For this review, take the finished solid that the model builds, in its own axes (mm). Round coordinates to 2 decimals unless told otherwise and drop trailing zeros. Loops run counter-clockwise (first coordinate to the right, second up) from the corner with the lowest first, then second, coordinate; pieces in that order, holes last.
1. Clearance check with flat-ended pins moving along their axes: pin 1 Ø7 at (x, y) = (59, 19) entering from +Z; pin 2 Ø1 at (x, z) = (68, -2.5) entering from +Y; pin 3 Ø3 at (y, z) = (51.5, -2.5) entering from +X. State where each tip first meets the part, or that it passes through.
2. Consider section A-A on x = 19. State the section outline as (y, z) points, then the cut area to 3 significant figures.
3. To check wall thickness, follow line 1 along Y through (x, z) = (19, 1.15); line 2 along Y through (x, z) = (16.5, 1.25); line 3 along X through (y, z) = (59.5, -1). State the ranges of each line that lie inside material, in increasing order.
4. Consider section B-B on z = 0.25. State the section outline as (x, y) points, then the cut area to 3 significant figures.
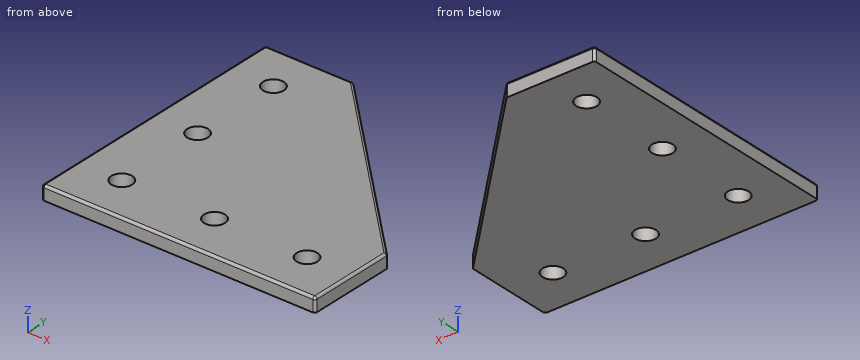
from build123d import *

# Parameters (mm, degrees)
SKETCH1_R           = 4.5
BOSS_EXTRUDE1_DEPTH = 3
FILLET1_R           = 1


with BuildPart() as part:
    # Sketch1 → Boss-Extrude1 (new, symmetric)
    with BuildSketch(Plane.XY):
        Polygon((0, 0), (0, 118), (38, 118), (118, 38), (118, 0), align=None)
        with Locations((19, 19)):
            Circle(SKETCH1_R, mode=Mode.SUBTRACT)
        with Locations((59, 19)):
            Circle(SKETCH1_R, mode=Mode.SUBTRACT)
        with Locations((99, 19)):
            Circle(SKETCH1_R, mode=Mode.SUBTRACT)
        with Locations((19, 59)):
            Circle(SKETCH1_R, mode=Mode.SUBTRACT)
        with Locations((19, 99)):
            Circle(SKETCH1_R, mode=Mode.SUBTRACT)
    extrude(amount=BOSS_EXTRUDE1_DEPTH, both=True)

    # Fillet1
    fillet1_edges = [part.edges().sort_by_distance(p)[0] for p in [
        (78, 78, 3),
        (19, 118, 3),
        (0, 59, 3),
        (59, 0, 3),
        (118, 19, 3),
        (0, 0, 0),
        (0, 118, 0),
        (38, 118, 0),
        (118, 38, 0),
        (118, 0, 0),
    ]]
    fillet(fillet1_edges, radius=FILLET1_R)


solid = part.part
Resolved:
1. pin 1: passes through
1. pin 2: stops at y = 88.5
1. pin 3: stops at x = 106
2. outline: (0, -3) - (14.5, -3) - (14.5, 3) - (1, 3) arc R1 ccw to (0, 2) - close; (23.5, -3) - (54.5, -3) - (54.5, 3) - (23.5, 3) - close; (63.5, -3) - (94.5, -3) - (94.5, 3) - (63.5, 3) - close; (103.5, -3) - (118, -3) - (118, 2) arc R1 ccw to (117, 3) - (103.5, 3) - close
2. area: 546 mm2
3. line 1: y = 0 to 14.5, 23.5 to 54.5, 63.5 to 94.5, 103.5 to 118
3. line 2: y = 0 to 15.26, 22.74 to 55.26, 62.74 to 95.26, 102.74 to 118
3. line 3: x = 0 to 14.53, 23.47 to 96.5
4. outline: (0, 1) arc R1 ccw to (1, 0) - (117, 0) arc R1 ccw to (118, 1) - (118, 37.59) arc R1 ccw to (117.71, 38.29) - (38.29, 117.71) arc R1 ccw to (37.59, 118) - (1, 118) arc R1 ccw to (0, 117) - close; hole circle Ø9 at (19, 19); hole circle Ø9 at (19, 59); hole circle Ø9 at (19, 99); hole circle Ø9 at (59, 19); hole circle Ø9 at (99, 19)
4. area: 10,400 mm2
